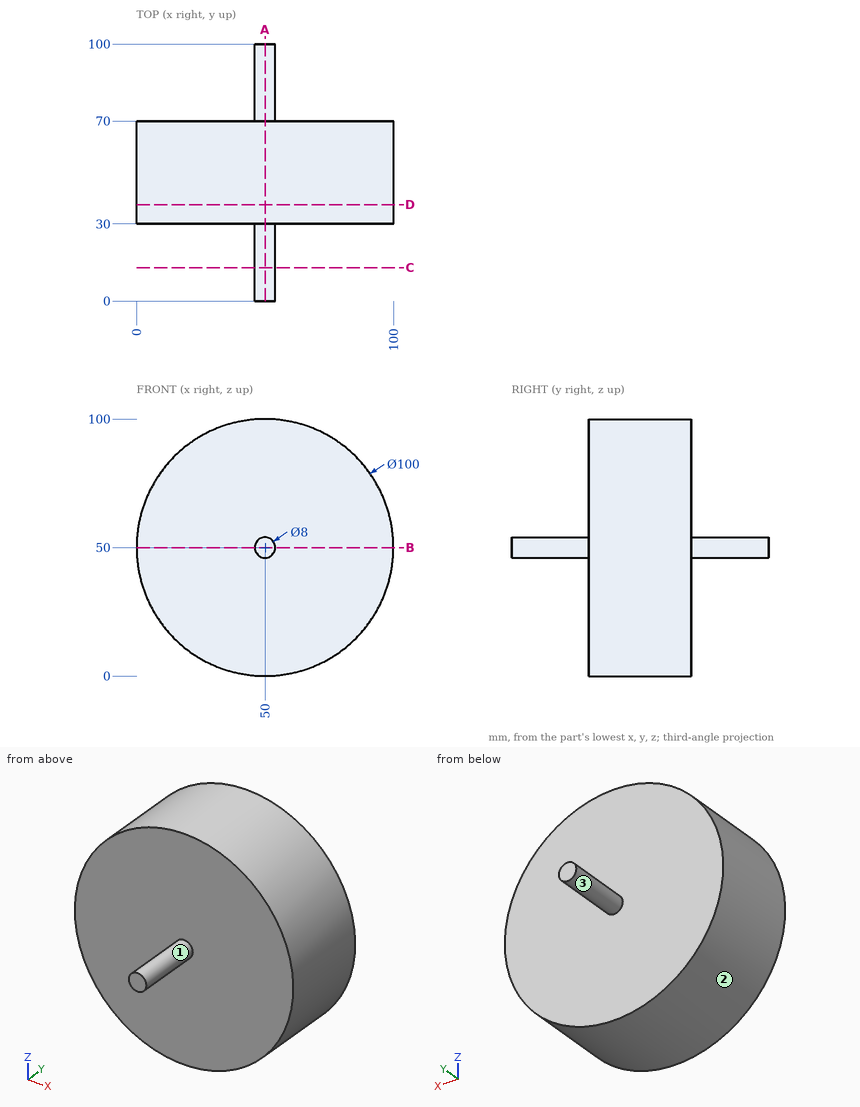
Geometry check sheet. Reference: drawing and pictorial views, mm from the part's lowest x, y, z. A direction names the side the tool comes from. Coordinates: 2 decimals unless noted, no trailing zeros. Write each loop counter-clockwise with the first axis right and the second up, starting at its lowest first coordinate (ties: lowest second). Pieces come first, ordered by that corner, then holes. Notation, with made-up numbers: (-0.75, 10.25) -> (36.25, 10.25) arc R20 cw to (36.25, 24.25) -> close; hole circle Ø1 at (77.25, -21.5). An arc over 180 degrees is marked (long way). One line per question, with ' | ' between items.
1. Set-up check for the marked faces 1, 2 and 3: record each of +Z, -Z, +X, -X, +Y, -Y from which the full face is reachable in a straight line by a thin tool's end or side.
Answers:
face 1: -Y | face 2: +Y, -Y | face 3: +Y
2. Cross-section at C-C on y = 13. Record the cut outline in (x, z), and give its area (3 significant figures).
Answers:
outline: circle Ø8 at (50, 50) | area: 50.3 mm²
3. Cross-section at D-D on y = 37.5. Record the cut outline in (x, z).
Answers:
outline: circle Ø100 at (50, 50)
4. Depth check by flat-ended pin: pin 1 Ø4 at (x, y) = (55, 69.5) entering from -Z; pin 2 Ø10 at (y, z) = (67, 63.5) entering from -X; pin 3 Ø5 at (x, y) = (82.5, 69) entering from -Z. Enter the tip coordinate at first touch or a pass-through.
Answers:
pin 1: stops at z = 0.09 | pin 2: stops at x = 0.73 | pin 3: stops at z = 10
5. Cross-section at B-B on z = 50. Record the cut outline in (x, y).
Answers:
outline: (0, 30) -> (46, 30) -> (46, 0) -> (54, 0) -> (54, 30) -> (100, 30) -> (100, 70) -> (54, 70) -> (54, 100) -> (46, 100) -> (46, 70) -> (0, 70) -> close
6. Thickness scan on probe 1 along Y at (x, z) = (28.5, 21); probe 2 along X at (y, z) = (32, 19); probe 3 along X at (y, z) = (49.5, 27). Record the ranges inside material, lowest first. Write a range as from..to.
Answers:
probe 1: y = 30..70 | probe 2: x = 10.77..89.23 | probe 3: x = 5.6..94.4
7. Cross-section at A-A on x = 50. Record the cut outline in (y, z), and give its area (3 significant figures).
Answers:
outline: (0, 46) -> (30, 46) -> (30, 0) -> (70, 0) -> (70, 46) -> (100, 46) -> (100, 54) -> (70, 54) -> (70, 100) -> (30, 100) -> (30, 54) -> (0, 54) -> close | area: 4,480 mm²
